Geometry: final body of the model. Coordinates: model frame, mm. Face numbers are marked on the shaded views. Round coordinates to 2 decimals unless told otherwise and drop trailing zeros. Loops run counter-clockwise (first coordinate to the right, second up) from the corner with the lowest first, then second, coordinate; pieces in that order, holes last. Notation, with made-up numbers: (-36, -24) -> (3, -24) arc R27 ccw to (3, 6) -> close; hole circle Ø9 at (12, -13). An arc over 180 degrees is marked (long way). Answer in a Markdown table with one row per item.
```python
from build123d import *

# Parameters (mm, degrees)
F0_R     = 105
F0_R_2   = 9.525
F0_R_3   = 2.38125
F1_DEPTH = 1.51892
F0_R_4   = 1.5875
F0_R_5   = 3.96875
F2_DEPTH = 6.35


with BuildPart() as f1:
    # F0 (on Top) → F1 (new body)
    with BuildSketch(Plane.XY):
        Circle(F0_R)
        with Locations((-25.8172762563, -87.9291171444)):
            Circle(F0_R_2, mode=Mode.SUBTRACT)
        with Locations((-69.2700381092, -59.9976934177)):
            Circle(F0_R_2, mode=Mode.SUBTRACT)
        with Locations((-83.3670032589, -38.0526498778)):
            Circle(F0_R_2, mode=Mode.SUBTRACT)
        with Locations((-49.5616522705, -77.0824494895)):
            Circle(F0_R_2, mode=Mode.SUBTRACT)
        with Locations((-30.5183343181, -62.8303570772)):
            Circle(F0_R_2, mode=Mode.SUBTRACT)
        with Locations((-0.2741651524, -69.8494619412)):
            Circle(F0_R_2, mode=Mode.SUBTRACT)
        with Locations((-15.4115002745, -47.472029452)):
            Circle(F0_R_2, mode=Mode.SUBTRACT)
        with Locations((-54.7328139874, -43.3974834872)):
            Circle(F0_R_2, mode=Mode.SUBTRACT)
        with Locations((-40.369082958, -29.3503843608)):
            Circle(F0_R_2, mode=Mode.SUBTRACT)
        with Locations((-20.3645865451, -20.3645865451)):
            Circle(F0_R_2, mode=Mode.SUBTRACT)
        with Locations((0, -91.640937332)):
            Circle(F0_R_2, mode=Mode.SUBTRACT)
        with Locations((25.8172762563, -87.9291171444)):
            Circle(F0_R_2, mode=Mode.SUBTRACT)
        with Locations((15.4312446271, -47.4656150309)):
            Circle(F0_R_2, mode=Mode.SUBTRACT)
        with Locations((30.5183343181, -62.8303570772)):
            Circle(F0_R_2, mode=Mode.SUBTRACT)
        with Locations((49.5431490419, -77.0943433599)):
            Circle(F0_R_2, mode=Mode.SUBTRACT)
        with Locations((0, -28.7998744842)):
            Circle(F0_R_2, mode=Mode.SUBTRACT)
        with Locations((20.3645865451, -20.3645865451)):
            Circle(F0_R_2, mode=Mode.SUBTRACT)
        with Locations((54.7328139874, -43.3974834872)):
            Circle(F0_R_2, mode=Mode.SUBTRACT)
        with Locations((40.3812875698, -29.3335905611)):
            Circle(F0_R_2, mode=Mode.SUBTRACT)
        with Locations((69.2556351005, -60.0143183075)):
            Circle(F0_R_2, mode=Mode.SUBTRACT)
        with Locations((83.3578672276, -38.0726590396)):
            Circle(F0_R_2, mode=Mode.SUBTRACT)
        with Locations((-90.7105821014, -13.0250408793)):
            Circle(F0_R_2, mode=Mode.SUBTRACT)
        with Locations((-90.7058866972, 13.0576993976)):
            Circle(F0_R_2, mode=Mode.SUBTRACT)
        with Locations((-68.1334048588, -15.3903100147)):
            Circle(F0_R_2, mode=Mode.SUBTRACT)
        with Locations((-68.0724721963, 15.6576188828)):
            Circle(F0_R_2, mode=Mode.SUBTRACT)
        with Locations((-83.3532974111, 38.082662798)):
            Circle(F0_R_2, mode=Mode.SUBTRACT)
        with Locations((-49.9109956825, -0.0207601598)):
            Circle(F0_R_2, mode=Mode.SUBTRACT)
        with Locations((-28.7998744842, 0)):
            Circle(F0_R_2, mode=Mode.SUBTRACT)
        with Locations((-40.3934851952, 29.3167916865)):
            Circle(F0_R_2, mode=Mode.SUBTRACT)
        with Locations((-54.5620548299, 43.6119785464)):
            Circle(F0_R_2, mode=Mode.SUBTRACT)
        with Locations((-20.3645865451, 20.3645865451)):
            Circle(F0_R_2, mode=Mode.SUBTRACT)
        with Locations((-69.2484320998, 60.0226294559)):
            Circle(F0_R_2, mode=Mode.SUBTRACT)
        with Locations((-49.5338963572, 77.1002886296)):
            Circle(F0_R_2, mode=Mode.SUBTRACT)
        with Locations((-30.2714865718, 62.9496592583)):
            Circle(F0_R_2, mode=Mode.SUBTRACT)
        with Locations((-15.4509863099, 47.4591923978)):
            Circle(F0_R_2, mode=Mode.SUBTRACT)
        with Locations((-25.8067234281, 87.9322149214)):
            Circle(F0_R_2, mode=Mode.SUBTRACT)
        Circle(F0_R_3, mode=Mode.SUBTRACT)
        with Locations((28.7998744842, 0)):
            Circle(F0_R_2, mode=Mode.SUBTRACT)
        with Locations((49.911, 0)):
            Circle(F0_R_2, mode=Mode.SUBTRACT)
        with Locations((0, 28.7998744842)):
            Circle(F0_R_2, mode=Mode.SUBTRACT)
        with Locations((20.3645865451, 20.3645865451)):
            Circle(F0_R_2, mode=Mode.SUBTRACT)
        with Locations((40.3812875698, 29.3335905611)):
            Circle(F0_R_2, mode=Mode.SUBTRACT)
        with Locations((54.5620548299, 43.6119785464)):
            Circle(F0_R_2, mode=Mode.SUBTRACT)
        with Locations((68.1334048588, -15.3903100147)):
            Circle(F0_R_2, mode=Mode.SUBTRACT)
        with Locations((68.0724721963, 15.6576188828)):
            Circle(F0_R_2, mode=Mode.SUBTRACT)
        with Locations((90.7074531384, -13.0468134127)):
            Circle(F0_R_2, mode=Mode.SUBTRACT)
        with Locations((90.7090182732, 13.0359272399)):
            Circle(F0_R_2, mode=Mode.SUBTRACT)
        with Locations((83.3624358436, 38.0626547328)):
            Circle(F0_R_2, mode=Mode.SUBTRACT)
        with Locations((15.4312446271, 47.4656150309)):
            Circle(F0_R_2, mode=Mode.SUBTRACT)
        with Locations((0, 69.85)):
            Circle(F0_R_2, mode=Mode.SUBTRACT)
        with Locations((30.2714865718, 62.9496592583)):
            Circle(F0_R_2, mode=Mode.SUBTRACT)
        with Locations((49.5524010131, 77.0883969799)):
            Circle(F0_R_2, mode=Mode.SUBTRACT)
        with Locations((0.0109981092, 91.640936672)):
            Circle(F0_R_2, mode=Mode.SUBTRACT)
        with Locations((25.8278287127, 87.9260181009)):
            Circle(F0_R_2, mode=Mode.SUBTRACT)
        with Locations((69.2628371036, 60.0060062947)):
            Circle(F0_R_2, mode=Mode.SUBTRACT)
    extrude(amount=F1_DEPTH)

    # F0 (on Top) → F2 (join)
    with BuildSketch(Plane.XY):
        with BuildLine():
            Line((-12.7, -108), (-12.7, -109.2644040848))
            ThreePointArc((-12.7, -109.2644040848), (0, -110), (12.7, -109.2644040848))
            Line((12.7, -109.2644040848), (12.7, -108))
            Line((12.7, -108), (-12.7, -108))
        make_face()
        with BuildLine():
            ThreePointArc((12.7, -109.2644040848), (82.1492544093, -73.1539472619), (110, 0))
            ThreePointArc((110, 0), (-73.1539472619, 82.1492544093), (-12.7, -109.2644040848))
            Line((-12.7, -109.2644040848), (-12.7, -108))
            Line((-12.7, -108), (12.7, -108))
            Line((12.7, -108), (12.7, -109.2644040848))
        make_face()
        Circle(F0_R, mode=Mode.SUBTRACT)
        with BuildLine():
            ThreePointArc((12.7, -109.2644040848), (0, -110), (-12.7, -109.2644040848))
            Line((-12.7, -109.2644040848), (-12.7, -141.3375))
            Line((-12.7, -141.3375), (12.7, -141.3375))
            Line((12.7, -141.3375), (12.7, -109.2644040848))
        make_face()
        with Locations((-8.73125, -120.7)):
            Circle(F0_R_4, mode=Mode.SUBTRACT)
        with Locations((0, -129.43125)):
            Circle(F0_R_4, mode=Mode.SUBTRACT)
        with Locations((0, -120.7)):
            Circle(F0_R_5, mode=Mode.SUBTRACT)
        with Locations((8.73125, -120.7)):
            Circle(F0_R_4, mode=Mode.SUBTRACT)
        with Locations((0, -111.96875)):
            Circle(F0_R_4, mode=Mode.SUBTRACT)
    extrude(amount=F2_DEPTH)


solid = f1.part
```
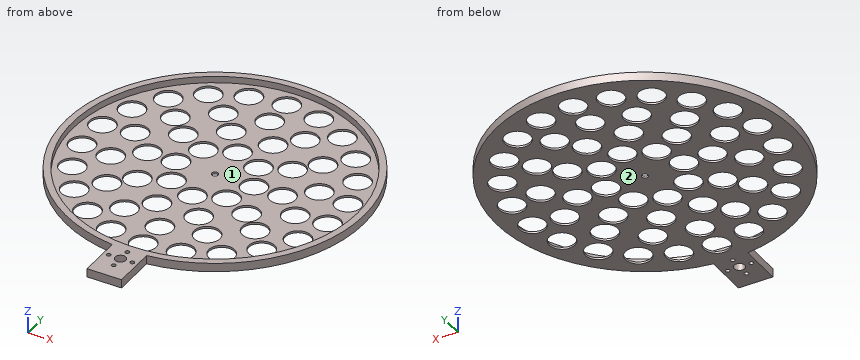
Item 1: Section query A-A, the plane x = 53. Output: boundary loops of the cut face in (y, z), and give its area (3 significant figures).
Ans:
| item | result |
|---|---|
| outline | (-96.39, 0) -> (-85.97, 0) -> (-85.97, 1.52) -> (-90.64, 1.52) -> (-90.64, 6.35) -> (-96.39, 6.35) -> close; (-68.22, 0) -> (-52.76, 0) -> (-52.76, 1.52) -> (-68.22, 1.52) -> close; (-34.03, 0) -> (-9.01, 0) -> (-9.01, 1.52) -> (-34.03, 1.52) -> close; (9.01, 0) -> (34.22, 0) -> (34.22, 1.52) -> (9.01, 1.52) -> close; (53.01, 0) -> (68.21, 0) -> (68.21, 1.52) -> (53.01, 1.52) -> close; (85.97, 0) -> (96.39, 0) -> (96.39, 6.35) -> (90.64, 6.35) -> (90.64, 1.52) -> (85.97, 1.52) -> close |
| area | 210 mm2 |
Item 2: Ray query, L1, parallel to X at y = -121, z = 5; L2, parallel to Y at x = 0, z = 4.75; L3, parallel to Y at x = -10, z = 4.75. Return the intervals inside material, ascending.
Ans:
| item | result |
|---|---|
| L1 | -12.7 to -10.29, -7.17 to -3.96, 3.96 to 7.17, 10.29 to 12.7 |
| L2 | -141.34 to -131.02, -127.84 to -124.67, -116.73 to -113.56, -110.38 to -105, 105 to 110 |
| L3 | -141.34 to -121.65, -119.75 to -104.52, 104.52 to 109.54 |
Item 3: First-contact query: P1, Ø1.5, axis at x = 46, z = 2.5, coming from the -Y side; P2, Ø1, axis at x = 61.5, z = 1.5, coming from the -Y side. Flat tips, straight axial feed; report the tip coordinate or a pass-through.
Ans:
| item | result |
|---|---|
| P1 | y = -100.26 |
| P2 | y = -91.54 |
Item 4: Section query B-B, the plane z = 5. Output: boundary loops of the cut face in (x, y) (1 decimal), and give its area (3 significant figures).
Ans:
| item | result |
|---|---|
| outline | (-12.7, -141.3) -> (12.7, -141.3) -> (12.7, -109.3) arc R110 ccw (long way) to (-12.7, -109.3) -> close; hole circle Ø210 at (0, 0); hole circle Ø3.2 at (-8.7, -120.7); hole circle Ø7.9 at (0, -120.7); hole circle Ø3.2 at (0, -129.4); hole circle Ø3.2 at (0, -112); hole circle Ø3.2 at (8.7, -120.7) |
| area | 4,100 mm2 |
Item 5: Mould query, pull axis X, two halves, no side actions, for the marked faces 1 and 2. Classes: released by +X, released by -X, zero draft, split by the parting line, or undercut.
Ans:
| item | result |
|---|---|
| face 1 | undercut |
| face 2 | zero draft |
